Input: part model. Units: mm. Frame: model coordinates. Face numbers are marked on the shaded views. A direction names the side the tool comes from. Round coordinates to 2 decimals unless told otherwise and drop trailing zeros. Loops run counter-clockwise (first coordinate to the right, second up) from the corner with the lowest first, then second, coordinate; pieces in that order, holes last. Notation, with made-up numbers: M 39.5,81 L 57.5,81 A9 ccw 57.5,96 Z; hole C -9,72 d9. An arc over 180 degrees is marked long. Use one line per item in the form item = value. Start each with the question number.
Q1. Mould query, pull axis Z, two halves, no side actions, for the marked faces 4, 5 and 6. Classes: pulls with the +Z half, pulls with the -Z half, needs draft (parallel to the pull), parting line crosses it, or undercut.
Q2. First-contact query: P1, Ø8, axis at x = -18, y = -6, coming from the +Z side; P2, Ø10, axis at x = -28, z = -9, coming from the -Y side; P3, Ø5.5, axis at x = -12, z = 9, coming from the +Y side; P4, Ø2, axis at y = -2, z = 0, coming from the -X side. Flat tips, straight axial feed; report the tip coordinate or a pass-through.
Q3. Section query C-C, the plane z = 0. Output: boundary loops of the cut face in (x, y).
Q4. Section query D-D, the plane x = 2.5. Output: boundary loops of the cut face in (y, z), and give its area (3 significant figures).
Q5. Section query A-A, the plane y = 4.75. Output: boundary loops of the cut face in (x, z), and give its area (3 significant figures).
Q6. Access query for the marked faces 1, 2 and 3. Directions: +Z, -Z, +X, -X, +Y, -Y. A direction counts if a zero-diameter tool reaches every point of the face in a straight line with its end or side. Return the directions, or none.
Q7. Ray query, line 1 along Z through (x, y) = (12, 3.6); line 2 along X through (y, z) = (0.5, 1); line 3 along Z through (x, y) = (23.5, -8.25). Return the intervals inside material, ascending.
Q8. Section query B-B, the plane x = -12. Output: boundary loops of the cut face in (y, z), and give its area (3 significant figures).
```python
from build123d import *

# Parameters (mm, degrees)
SKETCH1_R               = 1.75
SKETCH1_R_2             = 5
BOSS_EXTRUDE1_DEPTH     = 6
SKETCH2_R               = 3
SKETCH2_R_2             = 1.75
CUT_EXTRUDE1_DEPTH      = 3
CUT_EXTRUDE2_START      = -3
SKETCH3_R               = 8
SKETCH3_R_2             = 5
CUT_EXTRUDE2_DEPTH      = 3
SKETCH5_R               = 13.5
BOSS_EXTRUDE2_DEPTH     = 6
CUT_EXTRUDE3_DEPTH      = 47.983082062
CUT_EXTRUDE3_DEPTH_BACK = 47.983082062
SKETCH6_R               = 8
BOSS_EXTRUDE6_START     = -12
SKETCH9_R               = 11
SKETCH9_R_2             = 8
BOSS_EXTRUDE6_DEPTH     = 12
BOSS_EXTRUDE7_START     = 3
SKETCH10_R              = 11
SKETCH10_R_2            = 5
BOSS_EXTRUDE7_DEPTH     = 3
CHAMFER3_SIZE           = 2.5


with BuildPart() as part:
    # Sketch1 → Boss-Extrude1 (new body)
    with BuildSketch(Plane(origin=(0, 0, 0), x_dir=(1, 0, 0), z_dir=(0, 1, 0))):
        with BuildLine():
            Line((23.69, 13.5), (-31.1, 13.5))
            Line((-31.1, 13.5), (-31.1, 10.5))
            ThreePointArc((-31.1, 10.5), (-20.6, 0), (-31.1, -10.5))
            Line((-31.1, -10.5), (-31.1, -13.5))
            Line((-31.1, -13.5), (23.69, -13.5))
            Line((23.69, -13.5), (23.69, -11))
            ThreePointArc((23.69, -11), (34.69, 0), (23.69, 11))
            Line((23.69, 11), (23.69, 13.5))
        make_face()
        with Locations(Location((-12, -9, 0), (0, 0, 270))):
            Circle(SKETCH1_R, mode=Mode.SUBTRACT)
        with Locations(Location((12, -9, 0), (0, 0, 270))):
            Circle(SKETCH1_R, mode=Mode.SUBTRACT)
        with Locations(Location((-12, 9, 0), (0, 0, 270))):
            Circle(SKETCH1_R, mode=Mode.SUBTRACT)
        with Locations(Location((0, 0, 0), (0, 0, 270))):
            Circle(SKETCH1_R_2, mode=Mode.SUBTRACT)
        with Locations(Location((12, 9, 0), (0, 0, 270))):
            Circle(SKETCH1_R, mode=Mode.SUBTRACT)
        with Locations(Location((23.69, 0, 0), (0, 0, 270))):
            Circle(SKETCH1_R_2, mode=Mode.SUBTRACT)
    extrude(amount=BOSS_EXTRUDE1_DEPTH)

    # Sketch2 → Cut-Extrude1 (cut)
    # profile 1 of 4: a face of its own
    with BuildSketch(Plane.XZ):
        with Locations(Location((-12, -9, 0), (0, 0, 270))):
            Circle(SKETCH2_R)
        with Locations(Location((-12, -9, 0), (0, 0, 270))):
            Circle(SKETCH2_R_2, mode=Mode.SUBTRACT)
    # profile 2 of 4: a face of its own
    with BuildSketch(Plane.XZ):
        with Locations(Location((-12, 9, 0), (0, 0, 270))):
            Circle(SKETCH2_R)
        with Locations(Location((-12, 9, 0), (0, 0, 270))):
            Circle(SKETCH2_R_2, mode=Mode.SUBTRACT)
    # profile 3 of 4: a face of its own
    with BuildSketch(Plane.XZ):
        with Locations(Location((12, 9, 0), (0, 0, 270))):
            Circle(SKETCH2_R)
        with Locations(Location((12, 9, 0), (0, 0, 270))):
            Circle(SKETCH2_R_2, mode=Mode.SUBTRACT)
    # profile 4 of 4: a face of its own
    with BuildSketch(Plane.XZ):
        with Locations(Location((12, -9, 0), (0, 0, 270))):
            Circle(SKETCH2_R)
        with Locations(Location((12, -9, 0), (0, 0, 270))):
            Circle(SKETCH2_R_2, mode=Mode.SUBTRACT)
    extrude(amount=-CUT_EXTRUDE1_DEPTH, mode=Mode.SUBTRACT)

    # Sketch3 → Cut-Extrude2 (cut)
    # profile 1 of 2: a face of its own
    with BuildSketch(Plane(origin=(0, 6, 0), x_dir=(1, 0, 0), z_dir=(0, 1, 0)).offset(CUT_EXTRUDE2_START)):
        with Locations(Location((0, 0, 0), (0, 0, 270))):
            Circle(SKETCH3_R)
        with Locations(Location((0, 0, 0), (0, 0, 270))):
            Circle(SKETCH3_R_2, mode=Mode.SUBTRACT)
    # profile 2 of 2: a face of its own
    with BuildSketch(Plane(origin=(0, 6, 0), x_dir=(1, 0, 0), z_dir=(0, 1, 0)).offset(CUT_EXTRUDE2_START)):
        with Locations(Location((23.69, 0, 0), (0, 0, 270))):
            Circle(SKETCH3_R)
        with Locations(Location((23.69, 0, 0), (0, 0, 270))):
            Circle(SKETCH3_R_2, mode=Mode.SUBTRACT)
    extrude(amount=CUT_EXTRUDE2_DEPTH, mode=Mode.SUBTRACT)

    # Sketch5 → Boss-Extrude2 (add)
    with BuildSketch(Plane(origin=(0, 0, 0), x_dir=(1, 0, 0), z_dir=(0, 1, 0))):
        with Locations((-31.1, 0)):
            Circle(SKETCH5_R)
    extrude(amount=BOSS_EXTRUDE2_DEPTH)

    # Sketch6 → Cut-Extrude3 (cut, two sides: drawn at the far end of the back side and taken through both)
    with BuildSketch(Plane(origin=(0, 6, 0), x_dir=(1, 0, 0), z_dir=(0, 1, 0)).offset(-CUT_EXTRUDE3_DEPTH_BACK)):
        with Locations(Location((0, 0, 0), (0, 0, 270))):
            Circle(SKETCH6_R)
        with Locations(Location((23.69, 0, 0), (0, 0, 270))):
            Circle(SKETCH6_R)
    extrude(amount=CUT_EXTRUDE3_DEPTH + CUT_EXTRUDE3_DEPTH_BACK, mode=Mode.SUBTRACT)

    # Sketch9 → Boss-Extrude6 (add)
    # profile 1 of 2: a face of its own
    with BuildSketch(Plane(origin=(0, 0, 0), x_dir=(1, 0, 0), z_dir=(0, 1, 0)).offset(BOSS_EXTRUDE6_START)):
        with Locations(Location((0, 0, 0), (0, 0, 270))):
            Circle(SKETCH9_R)
        with Locations(Location((0, 0, 0), (0, 0, 270))):
            Circle(SKETCH9_R_2, mode=Mode.SUBTRACT)
    # profile 2 of 2: a face of its own
    with BuildSketch(Plane(origin=(0, 0, 0), x_dir=(1, 0, 0), z_dir=(0, 1, 0)).offset(BOSS_EXTRUDE6_START)):
        with BuildLine():
            ThreePointArc((23.69, 11), (12.69, 0), (23.69, -11))
            ThreePointArc((23.69, -11), (31.468174593, -7.778174593), (34.69, 0))
            ThreePointArc((34.69, 0), (31.468174593, 7.778174593), (23.69, 11))
        make_face()
        with Locations(Location((23.69, 0, 0), (0, 0, 270))):
            Circle(SKETCH9_R_2, mode=Mode.SUBTRACT)
    extrude(amount=BOSS_EXTRUDE6_DEPTH)

    # Sketch10 → Boss-Extrude7 (add)
    # profile 1 of 2: a face of its own
    with BuildSketch(Plane.XZ.offset(12).offset(BOSS_EXTRUDE7_START)):
        with Locations(Location((23.69, 0, 0), (0, 0, 270))):
            Circle(SKETCH10_R)
        with Locations(Location((23.69, 0, 0), (0, 0, 270))):
            Circle(SKETCH10_R_2, mode=Mode.SUBTRACT)
    # profile 2 of 2: a face of its own
    with BuildSketch(Plane.XZ.offset(12).offset(BOSS_EXTRUDE7_START)):
        with Locations(Location((0, 0, 0), (0, 0, 90))):
            Circle(SKETCH10_R)
        with Locations(Location((0, 0, 0), (0, 0, 270))):
            Circle(SKETCH10_R_2, mode=Mode.SUBTRACT)
    extrude(amount=-BOSS_EXTRUDE7_DEPTH)

    # Chamfer3
    # the kernel refuses this chamfer: 2.5 mm, written as the material it adds along each edge
    with BuildSketch(Plane(origin=(23.69, 0, 11), x_dir=(0.9912092295509808, 0, -0.13230367815352337), z_dir=(0, 1, 0))) as chamfer3_piece_1_section:
        with BuildLine():
            Line((2.910680919, 0), (-CHAMFER3_SIZE * 0.132303678154, -CHAMFER3_SIZE * 0.991209229551))
            Line((-CHAMFER3_SIZE * 0.132303678154, -CHAMFER3_SIZE * 0.991209229551), (0, 0))
            ThreePointArc((0, 0), (1.49552658, -0.096625069), (2.910680919, 0))
        make_face()
    chamfer3_piece_1 = extrude(amount=6, mode=Mode.PRIVATE)
    chamfer3_piece_1 = split(chamfer3_piece_1, bisect_by=Plane(origin=(23.69, 0, 13.5), z_dir=(0, 0, -1)), keep=Keep.TOP, mode=Mode.PRIVATE)
    add(chamfer3_piece_1)
    with BuildSketch(Plane(origin=(23.69, 0, -11), x_dir=(0, 0, -1), z_dir=(0, 1, 0))) as chamfer3_piece_2_section:
        with BuildLine():
            Line((CHAMFER3_SIZE, 0), (-0.385093792, -2.885093792))
            ThreePointArc((-0.385093792, -2.885093792), (-0.102088007, -1.495163601), (0, 0))
            Line((0, 0), (CHAMFER3_SIZE, 0))
        make_face()
    chamfer3_piece_2 = extrude(amount=6, mode=Mode.PRIVATE)
    chamfer3_piece_2 = split(chamfer3_piece_2, bisect_by=Plane(origin=(23.69, 0, -13.5), z_dir=(0, 0, 1)), keep=Keep.TOP, mode=Mode.PRIVATE)
    add(chamfer3_piece_2)


solid = part.part
```
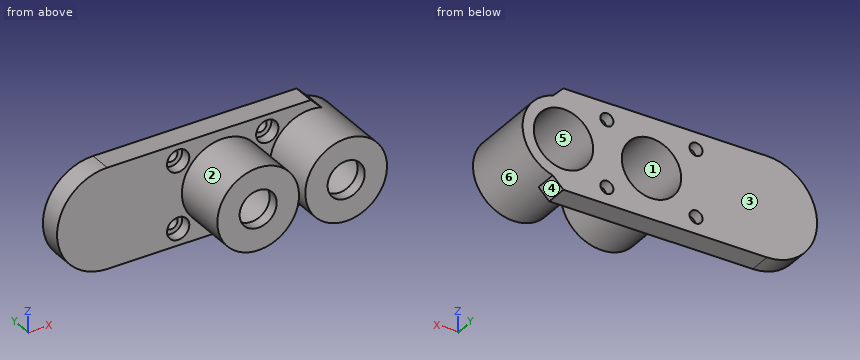
Results found:
q1.face_4 = pulls with the -Z half
q1.face_5 = undercut
q1.face_6 = parting line crosses it
q2.P1 = through
q2.P2 = 0
q2.P3 = 6
q2.P4 = -11
q3.outline = M -44.6,0 L -11,0 L -11,-15 L -5,-15 L -5,-12 L -8,-12 L -8,6 L -44.6,6 Z; M 5,-15 L 11,-15 L 11,0 L 12.69,0 L 12.69,-15 L 18.69,-15 L 18.69,-12 L 15.69,-12 L 15.69,6 L 8,6 L 8,-12 L 5,-12 Z; M 28.69,-15 L 34.69,-15 L 34.69,6 L 31.69,6 L 31.69,-12 L 28.69,-12 Z
q4.outline = M -15,-10.71 L 0,-10.71 L 0,-13.5 L 6,-13.5 L 6,-7.6 L -12,-7.6 L -12,-4.33 L -15,-4.33 Z; M -15,4.33 L -12,4.33 L -12,7.6 L 6,7.6 L 6,13.5 L 0,13.5 L 0,10.71 L -15,10.71 Z
q4.area = 184 mm²
q5.outline = M -31.1,-13.5 L 23.69,-13.5 L 26.58,-10.61 A11 ccw 26.58,10.61 L 23.69,13.5 L -31.1,13.5 A13.5 ccw Z; hole C -12,-9 d3.5; hole C -12,9 d3.5; hole C 0,0 d16; hole C 12,-9 d3.5; hole C 12,9 d3.5; hole C 23.69,0 d16
q5.area = 1,520 mm²
q6.face_1 = +Y
q6.face_2 = -Y
q6.face_3 = +Z, -Z, +X, -X, +Y
q7.line_1 = -13.5 to -10.75, -7.25 to 7.25, 10.75 to 13.5
q7.line_2 = -44.56 to -7.94, 7.94 to 15.75, 31.63 to 34.64
q7.line_3 = -11 to -8, 8 to 11
q8.outline = M 0,-13.5 L 6,-13.5 L 6,-10.75 L 3,-10.75 L 3,-12 L 0,-12 Z; M 0,-6 L 3,-6 L 3,-7.25 L 6,-7.25 L 6,7.25 L 3,7.25 L 3,6 L 0,6 Z; M 0,12 L 3,12 L 3,10.75 L 6,10.75 L 6,13.5 L 0,13.5 Z
q8.area = 105 mm²
